```python
from build123d import *

# Parameters (mm, degrees)
SKETCH_1_R          = 2
EXTRUDE_1_DEPTH     = 2
CUT_EXTRUDE_1_DEPTH = 73.508544139
FILLET_1_R          = 1


with BuildPart() as part:
    # 草图1 → 凸台-拉伸1 (new body)
    with BuildSketch(Plane(origin=(0, 0, 0), x_dir=(1, 0, 0), z_dir=(0, 1, 0))):
        with BuildLine():
            Line((-37.994784634, 24.205347356), (-44.62808047, 28.431222864))
            ThreePointArc((-44.62808047, 28.431222864), (-45.962279794, 30.395264974), (-45.451059851, 32.713929119))
            ThreePointArc((-45.451059851, 32.713929119), (0, 56), (45.451059851, 32.713929119))
            ThreePointArc((45.451059851, 32.713929119), (45.962279794, 30.395264974), (44.62808047, 28.431222864))
            Line((44.62808047, 28.431222864), (37.994784634, 24.205347356))
            ThreePointArc((37.994784634, 24.205347356), (0, 45.05), (-37.994784634, 24.205347356))
        make_face()
        with Locations(Location((37.123106012, 37.123106012, 0), (0, 0, 270))):
            Circle(SKETCH_1_R, mode=Mode.SUBTRACT)
        with Locations(Location((-37.123106012, 37.123106012, 0), (0, 0, 270))):
            Circle(SKETCH_1_R, mode=Mode.SUBTRACT)
    extrude(amount=EXTRUDE_1_DEPTH)

    # 草图2 → 切除-拉伸1 (cut, through all)
    with BuildSketch(Plane(origin=(0, 2, 0), x_dir=(1, 0, 0), z_dir=(0, 1, 0))):
        with BuildLine():
            ThreePointArc((-29.047558943, 41.980255114), (0, 51.05), (29.047558943, 41.980255114))
            ThreePointArc((29.047558943, 41.980255114), (31.350327582, 41.269688809), (33.643382893, 42.011001982))
            ThreePointArc((33.643382893, 42.011001982), (34.712414977, 42.617518513), (35.882608489, 42.993469365))
            ThreePointArc((35.882608489, 42.993469365), (0, 56), (-35.882608489, 42.993469365))
            ThreePointArc((-35.882608489, 42.993469365), (-34.712414977, 42.617518513), (-33.643382893, 42.011001982))
            ThreePointArc((-33.643382893, 42.011001982), (-31.350327582, 41.269688809), (-29.047558943, 41.980255114))
        make_face()
    extrude(amount=-CUT_EXTRUDE_1_DEPTH, mode=Mode.SUBTRACT)

    # 圆角1
    fillet_1_edges = [part.edges().sort_by_distance(p)[0] for p in [
        (-37.994784634, 1, -24.205347356),
        (37.994784634, 1, -24.205347356),
        (-35.882608489, 1, -42.993469365),
        (35.882608489, 1, -42.993469365),
    ]]
    fillet(fillet_1_edges, radius=FILLET_1_R)


solid = part.part
```
Build history of the part. All positions in model axes, mm. A direction names the side the tool comes from. Give positions to 0.01 mm unless a question says otherwise; leave off trailing zeros. Loops run counter-clockwise (first coordinate to the right, second up) from the corner with the lowest first, then second, coordinate; pieces in that order, holes last.
1) Drop a flat-ended pin along its axis: P1, Ø1, axis at x = 13, y = 0.5, coming from the +Z side. Give the stop position or say it passes through.
Values follow:
P1: stops at z = -42.98
2) Two-plate mould, pull along Z, no slides. Class faces 1 (the face through (-37.04, 0.99, -39.12)), 2 (the face through (0, 0, -46)), 3 (the face through (-41.232, 0.986, -37.894)), 4 (the face through (38.47, 0.99, -38.6)): released by +Z, released by -Z, zero draft, split by the parting line, or undercut.
Values follow:
face 1: undercut
face 2: zero draft
face 3: released by -Z
face 4: undercut
3) Band-saw the part on C-C on x = -16.5. List the corners of the cut face in (y, z), then the cut area to 3 significant figures.
Values follow:
outline: (0, -48.31) - (2, -48.31) - (2, -41.92) - (0, -41.92) - close
area: 12.8 mm2
4) 3-axis set-ups, long thin cutter, end or side, ignore diameter. For faces 5 (the face through (-34.468, 1.014, -42.504)), 6 (the face through (45.97, 0.99, -30.43)): which of +Z, -Z, +X, -X, +Y, -Y reach the whole face in a straight line?
Values follow:
face 5: -Z, +Y, -Y
face 6: +X, +Y, -Y
5) Probe line 1 along Z through (x, y) = (-37, 0.7); line 2 along X through (y, z) = (1.4, -33.25); line 3 along X through (y, z) = (0.6, -30.25). List the from-to ranges inside material, lowest first.
Values follow:
line 1: z = -42.04 to -39.12, -35.13 to -25.7
line 2: x = -45.06 to -30.4, 30.4 to 45.06
line 3: x = -45.93 to -33.38, 33.38 to 45.93
6) Band-saw the part on D-D on y = 0.4. State how many separate pieces and enclosed holes the cut face has, then the cut area to 3 significant figures.
Values follow:
separate pieces: 1
enclosed holes: 2
area: 726 mm2
7) Band-saw the part on A-A on z = -30.75. List the corners of the cut face in (x, y), then the cut area to 3 significant figures.
Values follow:
outline: (-46.01, 0) - (-32.92, 0) - (-32.92, 2) - (-46.01, 2) - close; (32.92, 0) - (46.01, 0) - (46.01, 2) - (32.92, 2) - close
area: 52.3 mm2
8) Band-saw the part on B-B on z = -37. List the corners of the cut face in (x, y).
Values follow:
outline: (-42.04, 0) - (-39.12, 0) - (-39.12, 2) - (-42.04, 2) - close; (-35.13, 0) - (-25.7, 0) - (-25.7, 2) - (-35.13, 2) - close; (25.7, 0) - (35.13, 0) - (35.13, 2) - (25.7, 2) - close; (39.12, 0) - (42.04, 0) - (42.04, 2) - (39.12, 2) - close
